from build123d import *

# Parameters (mm, degrees)
BOSS_EXTRUDE1_DEPTH = 20
SHELL4_T            = 2
FILLET2_R           = 5
CUT_EXTRUDE1_DEPTH  = 2


with BuildPart() as part:
    # Sketch2 → Boss-Extrude1 (new body)
    with BuildSketch(Plane(origin=(0, 0, 0), x_dir=(0, 0, -1), z_dir=(1, 0, 0))):
        with BuildLine():
            Line((-26.752483981, 30.914680653), (-20.431723376, -36.982479222))
            ThreePointArc((-20.431723376, -36.982479222), (-17.210158239, -43.447078966), (-10.474775424, -46.055555556))
            Line((-10.474775424, -46.055555556), (10.474775424, -46.055555556))
            ThreePointArc((10.474775424, -46.055555556), (17.210158239, -43.447078966), (20.431723376, -36.982479222))
            Line((20.431723376, -36.982479222), (26.752483981, 30.914680653))
            ThreePointArc((26.752483981, 30.914680653), (24.966551173, 37.606542438), (19.260935813, 41.532930539))
            ThreePointArc((19.260935813, 41.532930539), (0, 43.944444444), (-19.260935813, 41.532930539))
            ThreePointArc((-19.260935813, 41.532930539), (-24.966551173, 37.606542438), (-26.752483981, 30.914680653))
        make_face()
    extrude(amount=BOSS_EXTRUDE1_DEPTH)

    # Shell4
    shell4_openings = [part.faces().sort_by_distance(p)[0] for p in [
        (20, 0.813945533, 0),
    ]]
    offset(amount=SHELL4_T, openings=shell4_openings, kind=Kind.INTERSECTION)

    # Fillet2
    # the kernel refuses this fillet: 5 mm, written as the material it takes off along each edge
    with BuildSketch(Plane(origin=(-2, -48.055555556, 10.474775424), x_dir=(1, 0, 0), z_dir=(0, 0, -1))) as fillet2_piece_1:
        with BuildLine():
            CenterArc((FILLET2_R, -FILLET2_R), FILLET2_R, 90, 90)
            Line((0, -FILLET2_R), (0, 0))
            Line((0, 0), (FILLET2_R, 0))
        make_face()
    extrude(amount=20.949550847, mode=Mode.SUBTRACT)
    with BuildSketch(Plane(origin=(-2, -36.055555556, 10.474775424), x_dir=(0, -1, 0), z_dir=(0, 0, -1))) as fillet2_piece_2:
        with BuildLine():
            CenterArc((12 - FILLET2_R, -FILLET2_R), FILLET2_R, 0, 90)
            Line((12 - FILLET2_R, 0), (12, 0))
            Line((12, 0), (12, -FILLET2_R))
        make_face()
    revolve(axis=Axis((-2, -36.055555556, 10.474775424), (-1, 0, 0)), revolution_arc=84.681483972, mode=Mode.SUBTRACT)
    with BuildSketch(Plane(origin=(-2, 30.729295919, 28.743873571), x_dir=(1, 0, 0), z_dir=(0, -0.9956947951896508, -0.09269236663414848)), Plane(origin=(-2, -37.167863955, -22.423112966), x_dir=(1, 0, 0), z_dir=(0, 0.9956947951896508, -0.09269236663414848))) as fillet2_piece_3:
        with BuildLine():
            CenterArc((FILLET2_R, -FILLET2_R), FILLET2_R, 90, 90)
            Line((0, -FILLET2_R), (0, 0))
            Line((0, 0), (FILLET2_R, 0))
        make_face()
    extrude(amount=68.190734955, mode=Mode.SUBTRACT)
    with BuildSketch(Plane(origin=(-2, 31.841604319, 16.795536029), x_dir=(0, -0.09269236663414838, 0.9956947951896509), z_dir=(0, -0.9956947951896509, -0.09269236663414838))) as fillet2_piece_4:
        with BuildLine():
            CenterArc((12 - FILLET2_R, -FILLET2_R), FILLET2_R, 0, 90)
            Line((12 - FILLET2_R, 0), (12, 0))
            Line((12, 0), (12, -FILLET2_R))
        make_face()
    revolve(axis=Axis((-2, 31.841604319, 16.795536029), (-1, 0, 0)), revolution_arc=81.045656085, mode=Mode.SUBTRACT)
    with BuildSketch(Plane(origin=(-2, -34.180555556, 0), x_dir=(0, 0.9691326220109027, 0.2465399784097355), z_dir=(0, -0.2465399784097355, 0.9691326220109027))) as fillet2_piece_5:
        with BuildLine():
            CenterArc((80.125 - FILLET2_R, -FILLET2_R), FILLET2_R, 0, 90)
            Line((80.125 - FILLET2_R, 0), (80.125, 0))
            Line((80.125, 0), (80.125, -FILLET2_R))
        make_face()
    revolve(axis=Axis((-2, -34.180555556, 0), (-1, 0, 0)), revolution_arc=28.545719886, mode=Mode.SUBTRACT)
    with BuildSketch(Plane(origin=(-2, 31.841604319, -16.795536029), x_dir=(0, 0.9691326220109029, -0.24653997840973443), z_dir=(0, 0.24653997840973443, 0.9691326220109029))) as fillet2_piece_6:
        with BuildLine():
            CenterArc((12 - FILLET2_R, -FILLET2_R), FILLET2_R, 0, 90)
            Line((12 - FILLET2_R, 0), (12, 0))
            Line((12, 0), (12, -FILLET2_R))
        make_face()
    revolve(axis=Axis((-2, 31.841604319, -16.795536029), (-1, 0, 0)), revolution_arc=81.045656085, mode=Mode.SUBTRACT)
    with BuildSketch(Plane(origin=(-2, -36.055555556, -10.474775424), x_dir=(0, -0.09269236663414783, -0.9956947951896509), z_dir=(0, 0.9956947951896509, -0.09269236663414783))) as fillet2_piece_7:
        with BuildLine():
            CenterArc((12 - FILLET2_R, -FILLET2_R), FILLET2_R, 0, 90)
            Line((12 - FILLET2_R, 0), (12, 0))
            Line((12, 0), (12, -FILLET2_R))
        make_face()
    revolve(axis=Axis((-2, -36.055555556, -10.474775424), (-1, 0, 0)), revolution_arc=84.681483972, mode=Mode.SUBTRACT)

    # Sketch3 → Cut-Extrude1 (cut)
    with BuildSketch(Plane.XZ.offset(48.055555556)):
        with BuildLine():
            Line((20, -4.5), (20, 4.5))
            ThreePointArc((20, 4.5), (18.910791668, 4.274581528), (18.3, 3.345))
            Line((18.3, 3.345), (18.3, -3.345))
            ThreePointArc((18.3, -3.345), (18.910791668, -4.274581528), (20, -4.5))
        make_face()
    extrude(amount=-CUT_EXTRUDE1_DEPTH, mode=Mode.SUBTRACT)


solid = part.part
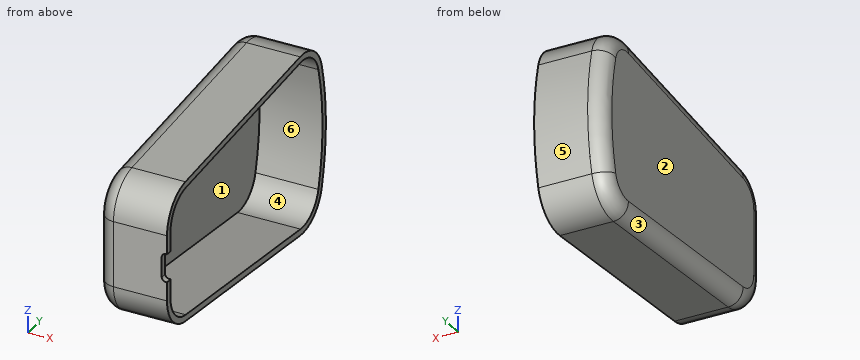
Here's how the part is built. I have some questions about the finished solid (model axes, mm). Face numbers are marked on the shaded views. A direction names the side the tool comes from. Give positions to 0.01 mm unless a question says otherwise; leave off trailing zeros. Loops run counter-clockwise (first coordinate to the right, second up) from the corner with the lowest first, then second, coordinate; pieces in that order, holes last. Notation, with made-up numbers: (29, 72) -> (56, 72) arc R24 ccw to (56, 86) -> close; hole circle Ø9 at (-2, 66). An arc over 180 degrees is marked (long way). One line per item, written item: value.
Q1. I'm going to push flat-ended pins straight in: pin 1 Ø10 at (x, y) = (13, -33) entering from -Z; pin 2 Ø6 at (x, y) = (14, 24) entering from -Z; pin 3 Ø5 at (y, z) = (2.5, -16.5) entering from +X. Where does each tip first touch, or does it pass through?
Answers follow:
pin 1: z = -23.28
pin 2: z = -28.4
pin 3: x = 0
Q2. Suppose I cut it at A-A on x = 13.75. Please give me the cut outline in (y, z) (3 decimals), then the cut area to 3 significant figures.
Answers follow:
outline: (-48.056, -10.475) arc R12 ccw to (-37.168, -22.423) -> (30.729, -28.744) arc R12 ccw to (43.471, -19.754) arc R80.125 ccw to (43.471, 19.754) arc R12 ccw to (30.729, 28.744) -> (-37.168, 22.423) arc R12 ccw to (-48.056, 10.475) -> close; hole (-46.056, -10.475) arc R10 ccw to (-36.982, -20.432) -> (30.915, -26.752) arc R10 ccw to (41.533, -19.261) arc R78.125 ccw to (41.533, 19.261) arc R10 ccw to (30.915, 26.752) -> (-36.982, 20.432) arc R10 ccw to (-46.056, 10.475) -> close
area: 521 mm^2
Q3. On a 3-axis mill with a long thin cutter (end or side, diameter ignored), from which of +Z, -Z, +X, -X, +Y, -Y can I reach the whole of each face in a straight line? I mean the marked faces 1 and 2. Say none if no direction works.
Answers follow:
face 1: +X
face 2: +Z, -Z, -X, +Y, -Y
Q4. If I drill on line 1 along X through (y, z) = (-12.5, -9.5); line 2 along Y through (x, z) = (8, -14.5); line 3 along Z through (x, y) = (3.5, -38), over which ranges is the centre line in solid material (lowest first)?
Answers follow:
line 1: -2 to 0
line 2: -47.36 to -45.21, 42.59 to 44.62
line 3: -22.32 to -20.28, 20.28 to 22.32
Q5. We'd pull the mould along Z, two halves only. Please class the marked faces 3, 4, 5 and 6: pulls with the +Z half, pulls with the -Z half, needs draft (parallel to the pull), parting line crosses it, or undercut.
Answers follow:
face 3: pulls with the -Z half
face 4: undercut
face 5: parting line crosses it
face 6: undercut
